from build123d import *

# Parameters (mm, degrees)
F1_DEPTH = 60
F3_D     = 25


with BuildPart() as f1:
    # F0 (on Right) → F1 (new body)
    with BuildSketch(Plane.YZ):
        Polygon((0, 30), (0, 0), (60, 0), (60, 60), (30, 60), align=None)
    extrude(amount=F1_DEPTH)

    # F3 (through all)
    with Locations(Plane.YZ.offset(60)):
        with Locations((32.045458, 26.022727)):
            Hole(F3_D / 2)


solid = f1.part
Design review of the part built by this model. Coordinates are the model's own, in mm. Give positions to 0.01 mm unless a question says otherwise; leave off trailing zeros. Write each loop counter-clockwise with the first axis right and the second up, starting at its lowest first coordinate (ties: lowest second). Pieces come first, ordered by that corner, then holes. Notation, with made-up numbers: M 6.5,22 L 47.5,22 A36 ccw 47.5,58 Z; hole C -33.5,87 d8. An arc over 180 degrees is marked long. Answer as a JSON object with one key per item and string values. Group by question number.
1) For line 1 along Y through (x, z) = (9.5, 25.5); line 2 along Z through (x, y) = (43.5, 40.5); line 3 along Y through (x, z) = (13, 19.5), list the stretches that pass through material, from the lowest coordinate up.
2) We need section B-B (z = 21.5). Give the boundary of the cut face in (x, y), and give its area (3 significant figures).
3) Clearance check with flat-ended pins moving along their axes: pin 1 Ø6 at (y, z) = (43.5, 45.5) entering from -X; pin 2 Ø1.5 at (x, z) = (37, 33.5) entering from -Y; pin 3 Ø1.5 at (x, z) = (38.5, 40) entering from -Y; pin 4 Ø4 at (x, y) = (6, 25.5) entering from +Z. State where each tip first meets the part, or that it passes through.
4) Mouldability with a two-part tool opening along Z and no side actions: class faces 1 (the face through (30, 15, 45)), 2 (the face through (30, 30, 0)), 3 (the face through (29.58, 41.26, 34.47)), 4 (the face through (60, 23, 37)) as released by +Z, released by -Z, zero draft, split by the parting line, or undercut.
5) We need section A-A (y = 34). Give the boundary of the cut face in (x, z), and give its area (3 significant figures).
6) We need section C-C (x = 22.5). Give the boundary of the cut face in (y, z), and give its area (3 significant figures).
7) We need section D-D (y = 18). Give the boundary of the cut face in (x, z).
Answer key:
{
 "1": {"line 1": "y = 0 to 19.56, 44.53 to 60", "line 2": "z = 0 to 16.82, 35.23 to 60", "line 3": "y = 0 to 21.38, 42.71 to 60"},
 "2": {"outline": "M 0,0 L 60,0 L 60,20.39 L 0,20.39 Z; M 0,43.7 L 60,43.7 L 60,60 L 0,60 Z", "area": "2,200 mm²"},
 "3": {"pin 1": "stops at x = 0", "pin 2": "stops at y = 2.75", "pin 3": "stops at y = 9.25", "pin 4": "stops at z = 57.5"},
 "4": {"face 1": "released by +Z", "face 2": "released by -Z", "face 3": "undercut", "face 4": "zero draft"},
 "5": {"outline": "M 0,0 L 60,0 L 60,13.68 L 0,13.68 Z; M 0,38.37 L 60,38.37 L 60,60 L 0,60 Z", "area": "2,120 mm²"},
 "6": {"outline": "M 0,0 L 60,0 L 60,60 L 30,60 L 0,30 Z; hole C 32.05,26.02 d25", "area": "2,660 mm²"},
 "7": {"outline": "M 0,0 L 60,0 L 60,48 L 0,48 Z"}
}
